Can you work these out from the model? Positions are in its coordinate system, mm. Face numbers are marked on the shaded views. Give positions to 0.01 mm unless a question says otherwise; leave off trailing zeros. Write each loop counter-clockwise with the first axis right and the second up, starting at its lowest first coordinate (ties: lowest second). Pieces come first, ordered by that corner, then holes.
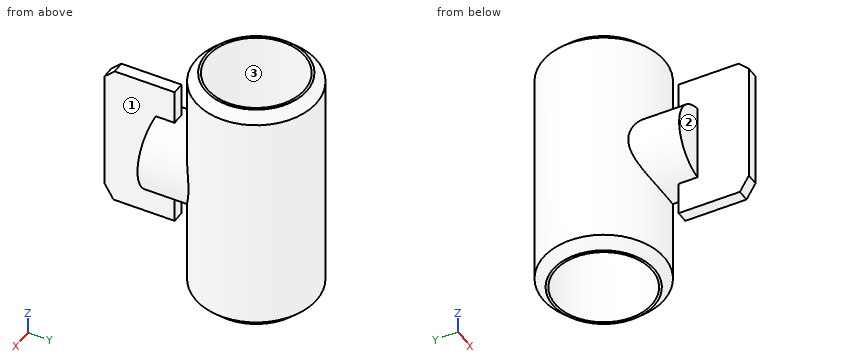
```python
from build123d import *

# Parameters (mm, degrees)
F0_R     = 12.5
F1_DEPTH = 50
F2_SIZE  = 2
F3_R     = 8.1072881944
F4_DEPTH = 20
F5_R     = 10
F6_DEPTH = 50.001
F8_DEPTH = 1.25


with BuildPart() as f1:
    # F0 (on Top) → F1 (new body)
    with BuildSketch(Plane.XY):
        Circle(F0_R)
    extrude(amount=F1_DEPTH)

    # F2
    f2_edges = [f1.edges().sort_by_distance(p)[0] for p in [
        (-12.5, 0, 50),
        (-12.5, 0, 0),
    ]]
    chamfer(f2_edges, length=F2_SIZE)

    # F3 (on Front) → F4 (join)
    with BuildSketch(Plane.XZ):
        with Locations((0, 24.8591881245)):
            Circle(F3_R)
    extrude(amount=F4_DEPTH)

    # F5 (on face) → F6 (cut, through all)
    with BuildSketch(Plane.XY.offset(50)):
        Circle(F5_R)
    extrude(amount=-F6_DEPTH, mode=Mode.SUBTRACT)

    # F7 (on Right) → F8 (join, symmetric)
    with BuildSketch(Plane.YZ):
        Polygon((-16.112501399, 40), (-28.4739788622, 40), (-30.5820492643, 38.0051359534), (-30.5820492643, 13.057355769), (-28.7352129817, 10), (-16.112501399, 10), align=None)
    extrude(amount=F8_DEPTH, both=True)


solid = f1.part
```
1) Please list where these lines run through material, in increasing order: L1, parallel to Y at x = 0, z = 38; L2, parallel to Y at x = 1, z = 38; L3, parallel to Y at x = 0, z = 22.
Values follow:
L1: y = -30.58 to -16.11, -12.5 to -10, 10 to 12.5
L2: y = -30.58 to -16.11, -12.46 to -9.95, 9.95 to 12.46
L3: y = -30.58 to -10, 10 to 12.5
2) If we mould it in two halves opening along Y, with no side actions, what happens to the marked faces 1, 2 and 3? For each: +Y half, -Y half, draft (parallel to the pull), parting line (faces both ways), or undercut.
Values follow:
face 1: draft
face 2: -Y half
face 3: undercut
3) Suppose I cut it at D-D on z = 23.5. Write out the boundary of the cut face in (x, y), plus the area to 3 significant figures.
Values follow:
outline: (-7.99, -20) - (-1.25, -20) - (-1.25, -30.58) - (1.25, -30.58) - (1.25, -20) - (7.99, -20) - (7.99, -9.61) arc R12.5 ccw (long way) to (-7.99, -9.61) - close; hole circle Ø20 at (0, 0)
area: 338 mm2
4) Suppose I cut it at A-A on y = 0. Write out the boundary of the cut face in (x, z).
Values follow:
outline: (-12.5, 2) - (-10.5, 0) - (-10, 0) - (-10, 50) - (-10.5, 50) - (-12.5, 48) - close; (10, 0) - (10.5, 0) - (12.5, 2) - (12.5, 48) - (10.5, 50) - (10, 50) - close
5) For pin 1 Ø2 at (x, z) = (-5.5, 24) entering from -Y; pin 2 Ø5 at (y, z) = (-14, 20.5) entering from -X; pin 3 Ø2 at (x, z) = (-2.5, 19) entering from +Y, each with a flat end and sliding along its axis, tell me the tip position at first contact or that it passes through.
Values follow:
pin 1: stops at y = -20
pin 2: stops at x = -7.89
pin 3: stops at y = 12.41
6) Suppose I cut it at B-B on x = 0. Write out the boundary of the cut face in (y, z).
Values follow:
outline: (-30.58, 13.06) - (-28.74, 10) - (-16.11, 10) - (-16.11, 16.75) - (-12.5, 16.75) - (-12.5, 2) - (-10.5, 0) - (-10, 0) - (-10, 50) - (-10.5, 50) - (-12.5, 48) - (-12.5, 32.97) - (-16.11, 32.97) - (-16.11, 40) - (-28.47, 40) - (-30.58, 38.01) - close; (10, 0) - (10.5, 0) - (12.5, 2) - (12.5, 48) - (10.5, 50) - (10, 50) - close
7) Suppose I cut it at C-C on z = 4.5. Write out the boundary of the cut face in (x, y).
Values follow:
outline: circle Ø25 at (0, 0); hole circle Ø20 at (0, 0)
